Input: part model. Units: mm. Frame: model coordinates. Face numbers are marked on the shaded views. A direction names the side the tool comes from. Give positions to 0.01 mm unless a question says otherwise; leave off trailing zeros. Loops run counter-clockwise (first coordinate to the right, second up) from the corner with the lowest first, then second, coordinate; pieces in that order, holes last.
from build123d import *

# Parameters (mm, degrees)
F0_W     = 100
F0_H     = 80
F0_R     = 15
F1_DEPTH = 50
F2_W     = 100
F2_H     = 20
F3_DEPTH = 50
F4_R     = 10
F5_DEPTH = 15


# Not quite as in the source:
# - a pattern or mirror of a feature is missing from the dataset's text; its kind, count and spacing are read off the source's solid


with BuildPart() as f1:
    # F0 (on Top) → F1 (new body)
    with BuildSketch(Plane.XY):
        Rectangle(F0_W, F0_H)
        Circle(F0_R, mode=Mode.SUBTRACT)
    extrude(amount=F1_DEPTH)

    # F2 (on Front) → F3 (cut)
    with BuildSketch(Plane.XZ):
        with Locations((0, 25)):
            Rectangle(F2_W, F2_H)
    extrude(amount=-F3_DEPTH, mode=Mode.SUBTRACT)

    # F4 (on face) → F5 (cut, through all)
    with BuildSketch(Plane.XY.offset(15)):
        with Locations((31.9020673633, 17.6108591259)):
            Circle(F4_R)
    f5 = extrude(amount=-F5_DEPTH, mode=Mode.SUBTRACT)

    # F5_copies: F5 across plane
    add(f5.mirror(Plane(origin=(0, 0, 0), x_dir=(0, 0, -1), z_dir=(-1, 0, 0))), mode=Mode.SUBTRACT)


solid = f1.part
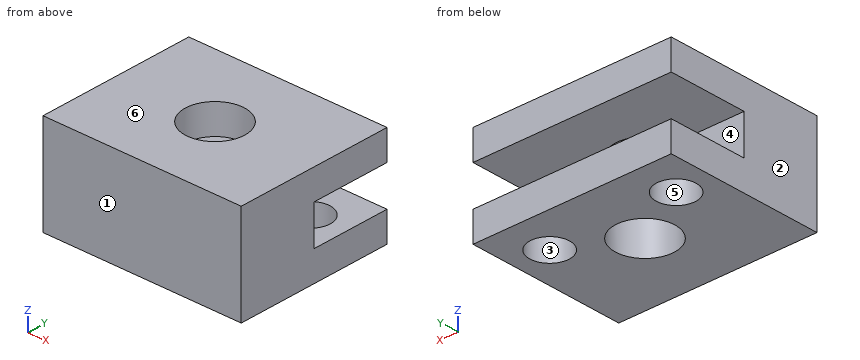
(1) Reachability of the marked faces 4, 5 and 6 from +Z, -Z, +X, -X, +Y, -Y: full face, straight path, thin tool, end or side. Return the list, or none.
Values follow:
face 4: +X, -X, +Y
face 5: -Z
face 6: +Z, +X, -X, +Y, -Y
(2) Cut plane B-B (y = 9). Return the cut outline in (x, z), and give its area (3 significant figures).
Values follow:
outline: (-50, 0) - (-36.99, 0) - (-36.99, 15) - (-50, 15) - close; (-50, 35) - (-12, 35) - (-12, 50) - (-50, 50) - close; (-26.82, 0) - (-12, 0) - (-12, 15) - (-26.82, 15) - close; (12, 0) - (26.82, 0) - (26.82, 15) - (12, 15) - close; (12, 35) - (50, 35) - (50, 50) - (12, 50) - close; (36.99, 0) - (50, 0) - (50, 15) - (36.99, 15) - close
area: 1,970 mm2
(3) Cut plane C-C (z = 6). Return the cut outline in (x, y), and give its area (3 significant figures).
Values follow:
outline: (-50, -40) - (50, -40) - (50, 40) - (-50, 40) - close; hole circle Ø20 at (-31.9, 17.61); hole circle Ø30 at (0, 0); hole circle Ø20 at (31.9, 17.61)
area: 6,660 mm2
(4) Cut plane D-D (x = 37.5). Return the cut outline in (y, z), and give its area (3 significant figures).
Values follow:
outline: (-40, 0) - (9.32, 0) - (9.32, 15) - (0, 15) - (0, 35) - (40, 35) - (40, 50) - (-40, 50) - close; (25.9, 0) - (40, 0) - (40, 15) - (25.9, 15) - close
area: 2,950 mm2
(5) Ray query, probe 1 along Y at (x, z) = (0.5, 42); probe 2 along Z at (x, y) = (17, 31); probe 3 along X at (y, z) = (22, 5). Return the intervals inside material, ascending.
Values follow:
probe 1: y = -40 to -14.99, 14.99 to 40
probe 2: z = 0 to 15, 35 to 50
probe 3: x = -50 to -40.89, -22.92 to 22.92, 40.89 to 50
(6) Pin query (flat end, axial travel): pin 1 Ø6 at (x, z) = (31.5, 27) entering from +Y. Return the tip coordinate at first contact, or that it passes through.
Values follow:
pin 1: stops at y = 0
(7) Cut plane A-A (x = 0). Return the cut outline in (y, z).
Values follow:
outline: (-40, 0) - (-15, 0) - (-15, 50) - (-40, 50) - close; (15, 0) - (40, 0) - (40, 15) - (15, 15) - close; (15, 35) - (40, 35) - (40, 50) - (15, 50) - close
(8) Mould query, pull axis Y, two halves, no side actions, for the marked faces 1, 2 and 3. Classes: +Y half, -Y half, draft (parallel to the pull), parting line (faces both ways), or undercut.
Values follow:
face 1: -Y half
face 2: draft
face 3: undercut
